Geometry check sheet. Reference: the model listing, model coordinates, mm. Face numbers are marked on the shaded views. Give positions to 0.01 mm unless a question says otherwise; leave off trailing zeros. Write each loop counter-clockwise with the first axis right and the second up, starting at its lowest first coordinate (ties: lowest second). Pieces come first, ordered by that corner, then holes. Notation, with made-up numbers: (-19, 25) -> (33, 25) arc R22 ccw to (33, 33) -> close; hole circle Ø3 at (-15.75, 78). An arc over 180 degrees is marked (long way). Write item = value, one per line. Start each with the question number.
1. Mould release check, pull along X, two halves, no side actions. Record for the marked faces 1, 2 and 3: pulls with the +X half, pulls with the -X half, needs draft (parallel to the pull), parting line crosses it, or undercut.
2. Thickness scan on line 1 along Z through (x, y) = (5, 22.5); line 2 along Y through (x, z) = (11, 1.75); line 3 along Y through (x, z) = (18, 2). Record the ranges inside material, lowest first.
3. Depth check by flat-ended pin: P1, Ø12, axis at x = 9.5, y = 14.5, coming from the -Z side; P2, Ø1.5, axis at y = 18, z = 4, coming from the -X side; P3, Ø3, axis at x = 29, z = 4, coming from the +Y side. Enter the tip coordinate at first touch or a pass-through.
4. Cross-section at B-B, the plane x = 6. Record the cut outline in (y, z) (3 decimals), plus the area to 3 significant figures.
5. Cross-section at A-A, the plane z = 2.25. Record the cut outline in (x, y), plus the area to 3 significant figures.
6. Cross-section at C-C, the plane z = -2. Record the cut outline in (x, y).
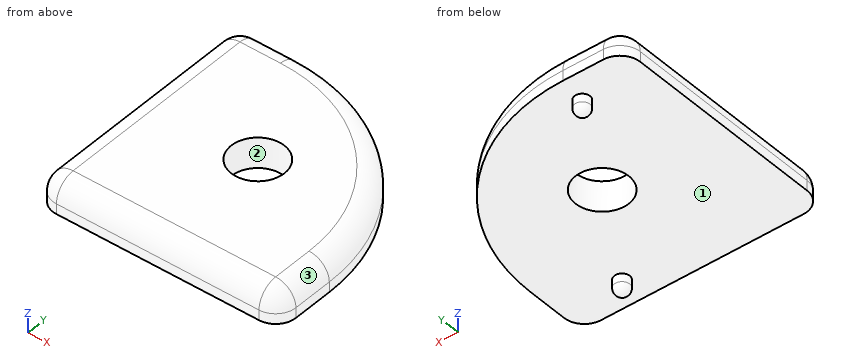
```python
from build123d import *

# Parameters (mm, degrees)
SKETCH1_R      = 4.1656
EXTRUDE1_DEPTH = 4.7752
FILLET1_R      = 3.175
SKETCH2_R      = 1.2065
EXTRUDE2_DEPTH = 2.4892
FILLET2_R      = 1.2065


with BuildPart() as part:
    # Sketch1 → Extrude1 (new body)
    with BuildSketch(Plane.XY):
        with BuildLine():
            Line((39.944028629, 9.505986328), (39.944028629, 15.855986328))
            ThreePointArc((39.944028629, 15.855986328), (31.574604902, 36.0615626), (11.369028629, 44.430986328))
            Line((11.369028629, 44.430986328), (5.019028629, 44.430986328))
            ThreePointArc((5.019028629, 44.430986328), (2.773964599, 43.501050358), (1.844028629, 41.255986328))
            Line((1.844028629, 41.255986328), (1.844028629, 9.505986328))
            ThreePointArc((1.844028629, 9.505986328), (2.773964599, 7.260922298), (5.019028629, 6.330986328))
            Line((5.019028629, 6.330986328), (36.769028629, 6.330986328))
            ThreePointArc((36.769028629, 6.330986328), (39.014092659, 7.260922298), (39.944028629, 9.505986328))
        make_face()
        with Locations((20.894028629, 25.380986328)):
            Circle(SKETCH1_R, mode=Mode.SUBTRACT)
    extrude(amount=EXTRUDE1_DEPTH)

    # Fillet1
    fillet1_edges = [part.edges().sort_by_distance(p)[0] for p in [
        (39.944028629, 12.680986328, 4.7752),
        (31.574604902, 36.0615626, 4.7752),
        (8.194028629, 44.430986328, 4.7752),
        (2.773964599, 43.501050358, 4.7752),
        (1.844028629, 25.380986328, 4.7752),
        (2.773964599, 7.260922298, 4.7752),
        (20.894028629, 6.330986328, 4.7752),
        (39.014092659, 7.260922298, 4.7752),
    ]]
    fillet(fillet1_edges, radius=FILLET1_R)

    # Sketch2 → Extrude2 (add)
    with BuildSketch(Plane(origin=(0, 0, 0), x_dir=(-1, 0, 0), z_dir=(0, 0, -1))):
        with Locations(Location((-29.911028629, 10.648986328, 0), (0, 0, 180))):
            Circle(SKETCH2_R)
        with Locations(Location((-11.877028629, 40.112986328, 0), (0, 0, 180))):
            Circle(SKETCH2_R)
    extrude(amount=EXTRUDE2_DEPTH)

    # Fillet2
    fillet2_edges = [part.edges().sort_by_distance(p)[0] for p in [
        (28.704528629, 10.648986328, -2.4892),
        (10.670528629, 40.112986328, -2.4892),
    ]]
    fillet(fillet2_edges, radius=FILLET2_R)


solid = part.part
```
Answers:
q1.face_1 = needs draft
q1.face_2 = undercut
q1.face_3 = pulls with the +X half
q2.line_1 = 0 to 4.78
q2.line_2 = 6.33 to 44.43
q2.line_3 = 6.36 to 22.38, 28.38 to 43.62
q3.P1 = 0
q3.P2 = 2.31
q3.P3 = 38.78
q4.outline = (6.331, 0) -> (44.431, 0) -> (44.431, 1.6) arc R3.175 ccw to (41.256, 4.775) -> (9.506, 4.775) arc R3.175 ccw to (6.331, 1.6) -> close
q4.area = 178 mm^2
q5.outline = (1.91, 9.51) arc R3.11 ccw to (5.02, 6.4) -> (36.77, 6.4) arc R3.11 ccw to (39.88, 9.51) -> (39.88, 15.86) arc R28.51 ccw to (11.37, 44.36) -> (5.02, 44.36) arc R3.11 ccw to (1.91, 41.26) -> close; hole circle Ø8.33 at (20.89, 25.38)
q5.area = 1,210 mm^2
q6.outline = circle Ø1.94 at (11.88, 40.11); circle Ø1.94 at (29.91, 10.65)
